```python
from build123d import *

# Parameters (mm, degrees)
EXTRUDE_1_DEPTH        = 250
SKETCH_2_R             = 1.25
CUT_EXTRUDE_3_DEPTH    = 251.074488903
PATTERN_LINEAR_1_COUNT = 5
PATTERN_LINEAR_1_PITCH = 15


with BuildPart() as part:
    # 草图1 → 凸台-拉伸1 (new body)
    with BuildSketch(Plane(origin=(0, 0, 0), x_dir=(1, 0, 0), z_dir=(0, 1, 0))):
        Polygon((-3.5, 1.5), (-1.5, 1), (-3.5, 0.5), (-3.5, -2.5), (3.5, -2.5), (3.5, 0.5), (1.5, 1), (3.5, 1.5), (3.5, 2.5), (-3.5, 2.5), align=None)
    extrude(amount=EXTRUDE_1_DEPTH)

    # 草图2 → 切除-拉伸3 (cut, through all)
    with BuildSketch(Plane(origin=(0, 0, -2.5), x_dir=(-1, 0, 0), z_dir=(0, 0, -1))):
        with Locations((0, 245)):
            Circle(SKETCH_2_R)
    cut_extrude_3 = extrude(amount=-CUT_EXTRUDE_3_DEPTH, mode=Mode.SUBTRACT)

    # 阵列(线性)1: 切除-拉伸3 ×5
    with Locations(*[(0, -i * PATTERN_LINEAR_1_PITCH, 0) for i in range(1, PATTERN_LINEAR_1_COUNT)]):
        add(cut_extrude_3, mode=Mode.SUBTRACT)


solid = part.part
```
CAD build for the part. Positions are in the model's coordinates, mm. Round coordinates to 2 decimals unless told otherwise and drop trailing zeros. Write each loop counter-clockwise with the first axis right and the second up, starting at its lowest first coordinate (ties: lowest second). Pieces come first, ordered by that corner, then holes.
Item 1: Drill centre lines: L1, parallel to Y at x = 0, z = 1.35; L2, parallel to X at y = 185, z = 0.15; L3, parallel to Y at x = -0.75, z = 1.85. Where is each one in solid material? Low to high.
Filled in:
L1: y = 0 to 183.75, 186.25 to 198.75, 201.25 to 213.75, 216.25 to 228.75, 231.25 to 243.75, 246.25 to 250
L2: x = -3.5 to -1.25, 1.25 to 3.5
L3: y = 0 to 184, 186 to 199, 201 to 214, 216 to 229, 231 to 244, 246 to 250
Item 2: Band-saw the part on A-A on x = 0. Write the cut outline in (y, z), then the cut area to 3 significant figures.
Filled in:
outline: (0, -2.5) - (183.75, -2.5) - (183.75, 2.5) - (0, 2.5) - close; (186.25, -2.5) - (198.75, -2.5) - (198.75, 2.5) - (186.25, 2.5) - close; (201.25, -2.5) - (213.75, -2.5) - (213.75, 2.5) - (201.25, 2.5) - close; (216.25, -2.5) - (228.75, -2.5) - (228.75, 2.5) - (216.25, 2.5) - close; (231.25, -2.5) - (243.75, -2.5) - (243.75, 2.5) - (231.25, 2.5) - close; (246.25, -2.5) - (250, -2.5) - (250, 2.5) - (246.25, 2.5) - close
area: 1,190 mm2
Item 3: Drop a flat-ended pin along its axis: pin 1 Ø3 at (x, z) = (-3, 2) entering from -Y. Give the stop position or say it passes through.
Filled in:
pin 1: stops at y = 0
Item 4: Band-saw the part on B-B on y = 42. Write the cut outline in (x, z), then the cut area to 3 significant figures.
Filled in:
outline: (-3.5, -2.5) - (3.5, -2.5) - (3.5, -1.5) - (1.5, -1) - (3.5, -0.5) - (3.5, 2.5) - (-3.5, 2.5) - (-3.5, -0.5) - (-1.5, -1) - (-3.5, -1.5) - close
area: 33.0 mm2
